Here's how the part is built. I have some questions about the finished solid (model axes, mm). Face numbers are marked on the shaded views. A direction names the side the tool comes from. Coordinates: 2 decimals unless noted, no trailing zeros. Write each loop counter-clockwise with the first axis right and the second up, starting at its lowest first coordinate (ties: lowest second). Pieces come first, ordered by that corner, then holes.
Item 1: I want a section at B-B (z = 113.5). Please give me the cut outline in (x, y), and give its area (3 significant figures).
Item 2: If we mould it in two halves opening along Z, with no side actions, what happens to the marked faces 3 and 4? For each: pulls with the +Z half, pulls with the -Z half, needs draft (parallel to the pull), parting line crosses it, or undercut.
Item 3: I want a section at A-A (x = 6.5). Please give me the cut outline in (y, z), and give its area (3 significant figures).
Item 4: I want a section at C-C (y = -5). Please give me the cut outline in (x, z) (3 decimals).
Item 5: I'm going to push flat-ended pins straight in: P1, Ø8, axis at x = -12.5, y = -5, coming from the -Z side; P2, Ø1.5, axis at x = -13.5, z = 116.5, coming from the +Y side; P3, Ø10.5, axis at x = 3.5, z = 127, coming from the +Y side; P4, Ø1.3, axis at y = -1, z = 110, coming from the -X side. Where does each tip first touch, or does it pass through?
Item 6: Please list where these lines run through material, in increasing order: line 1 (Z direction, x = -8.68, y = -11.1); line 2 (Y direction, x = -6, z = 143); line 3 (X direction, y = -0.5, z = 44.5).
Item 7: For the marked faces 1 and 2, which set-ups out of +Z, -Z, +X, -X, +Y, -Y let a thin tool reach every point of the face, with its end or its side?
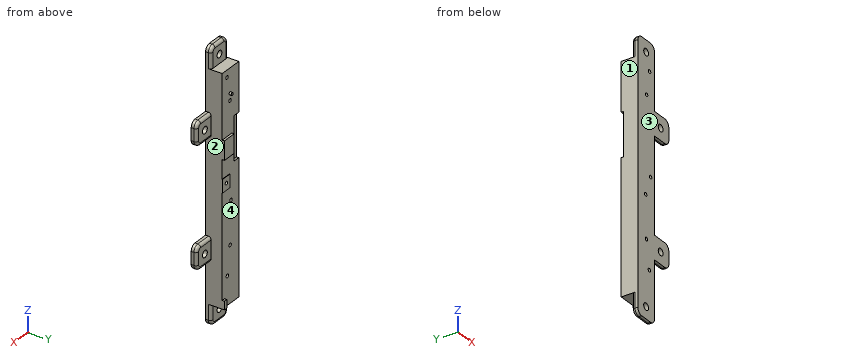
from build123d import *

# Parameters (mm, degrees)
SKETCH1_R           = 1
SKETCH1_R_2         = 1.25
SKETCH1_W           = 10.1
SKETCH1_H           = 13.47
SKETCH1_W_2         = 2.5
SKETCH1_H_2         = 6
SKETCH1_W_3         = 5.08
SKETCH1_H_3         = 31.36
BOSS_EXTRUDE1_DEPTH = 12
SKETCH1_3_W         = 10.1
SKETCH1_3_H         = 13.47
SKETCH1_3_W_2       = 2.5
SKETCH1_3_H_2       = 6
SKETCH1_3_R         = 1
BOSS_EXTRUDE2_DEPTH = 1.6
SKETCH1_4_W         = 5.08
SKETCH1_4_H         = 31.36
CUT_EXTRUDE1_DEPTH  = 1.6
BOSS_EXTRUDE3_START = 0.3
SKETCH2_W           = 7.8
SKETCH2_H           = 9.45
SKETCH2_R           = 1.25
BOSS_EXTRUDE3_DEPTH = 0.3
SKETCH3_W           = 17.3
SKETCH3_H           = 4
BOSS_EXTRUDE4_DEPTH = 15
SKETCH4_W           = 17.3
SKETCH4_H           = 4
BOSS_EXTRUDE5_DEPTH = 15
SKETCH5_W           = 17
SKETCH5_H           = 4
BOSS_EXTRUDE6_DEPTH = 15
FILLET1_R           = 4
FILLET2_R           = 2
CUT_EXTRUDE2_REACH  = 180.5
SKETCH6_R           = 2.5


with BuildPart() as part:
    # Sketch1 → Boss-Extrude1 (new body)
    # profile 1 of 5: a face of its own
    with BuildSketch(Plane(origin=(0, 0, 0), x_dir=(1, 0, 0), z_dir=(0, 1, 0))):
        Polygon((-2.5, -6), (-2.5, 0), (-17.3, 0), (-17.3, -96.08), (-12.22, -96.08), (-12.22, -127.44), (-17.3, -127.44), (-17.3, -162.4), (0, -162.4), (0, -116.51), (-10.1, -116.51), (-10.1, -103.04), (0, -103.04), (0, -6), align=None)
        with Locations((-8.115, -144.895)):
            Circle(SKETCH1_R, mode=Mode.SUBTRACT)
        with Locations(Location((-5.05, -157.28, 0), (0, 0, 270))):
            Circle(SKETCH1_R_2, mode=Mode.SUBTRACT)
        with Locations(Location((-8.115, -139.85, 0), (0, 0, 270))):
            Circle(SKETCH1_R_2, mode=Mode.SUBTRACT)
        with Locations(Location((-3.95, -85.02, 0), (0, 0, 270))):
            Circle(SKETCH1_R_2, mode=Mode.SUBTRACT)
        with Locations(Location((-9.115, -70.745, 0), (0, 0, 270))):
            Circle(SKETCH1_R_2, mode=Mode.SUBTRACT)
        with Locations(Location((-8.25, -40.21, 0), (0, 0, 270))):
            Circle(SKETCH1_R_2, mode=Mode.SUBTRACT)
        with Locations(Location((-5.3, -20.3, 0), (0, 0, 270))):
            Circle(SKETCH1_R_2, mode=Mode.SUBTRACT)
    # profile 2 of 5: a face of its own
    with BuildSketch(Plane(origin=(0, 0, 0), x_dir=(1, 0, 0), z_dir=(0, 1, 0))):
        with Locations((-5.05, -109.775)):
            Rectangle(SKETCH1_W, SKETCH1_H)
    # profile 3 of 5: a face of its own
    with BuildSketch(Plane(origin=(0, 0, 0), x_dir=(1, 0, 0), z_dir=(0, 1, 0))):
        with Locations((-1.25, -3)):
            Rectangle(SKETCH1_W_2, SKETCH1_H_2)
    # profile 4 of 5: a face of its own
    with BuildSketch(Plane(origin=(0, 0, 0), x_dir=(1, 0, 0), z_dir=(0, 1, 0))):
        with Locations((-14.76, -111.76)):
            Rectangle(SKETCH1_W_3, SKETCH1_H_3)
    # profile 5 of 5: a face of its own
    with BuildSketch(Plane(origin=(0, 0, 0), x_dir=(1, 0, 0), z_dir=(0, 1, 0))):
        with Locations((-8.115, -144.895)):
            Circle(SKETCH1_R)
    extrude(amount=-BOSS_EXTRUDE1_DEPTH)

    # Sketch1<3> → Boss-Extrude2 (add)
    with BuildSketch(Plane(origin=(0, 0, 0), x_dir=(1, 0, 0), z_dir=(0, 1, 0))):
        with Locations((-5.05, -109.775)):
            Rectangle(SKETCH1_3_W, SKETCH1_3_H)
        with Locations((-1.25, -3)):
            Rectangle(SKETCH1_3_W_2, SKETCH1_3_H_2)
        with Locations(Location((-8.115, -144.895, 0), (0, 0, 270))):
            Circle(SKETCH1_3_R)
    extrude(amount=BOSS_EXTRUDE2_DEPTH)

    # Sketch1<4> → Cut-Extrude1 (cut)
    with BuildSketch(Plane(origin=(0, 0, 0), x_dir=(1, 0, 0), z_dir=(0, 1, 0))):
        with Locations((-14.76, -111.76)):
            Rectangle(SKETCH1_4_W, SKETCH1_4_H)
    extrude(amount=-CUT_EXTRUDE1_DEPTH, mode=Mode.SUBTRACT)

    # Sketch2 → Boss-Extrude3 (add)
    with BuildSketch(Plane(origin=(0, 0, 0), x_dir=(1, 0, 0), z_dir=(0, 1, 0)).offset(BOSS_EXTRUDE3_START)):
        with Locations((-3.9, -84.835)):
            Rectangle(SKETCH2_W, SKETCH2_H)
        with Locations(Location((-3.95, -85.02, 0), (0, 0, 270))):
            Circle(SKETCH2_R, mode=Mode.SUBTRACT)
    extrude(amount=-BOSS_EXTRUDE3_DEPTH)

    # Sketch3 → Boss-Extrude4 (add)
    with BuildSketch(Plane.XY.offset(162.4)):
        with Locations((-8.65, -10)):
            Rectangle(SKETCH3_W, SKETCH3_H)
    extrude(amount=BOSS_EXTRUDE4_DEPTH)

    # Sketch4 → Boss-Extrude5 (add)
    with BuildSketch(Plane(origin=(0, 0, 0), x_dir=(-1, 0, 0), z_dir=(0, 0, -1))):
        with Locations((8.65, -10)):
            Rectangle(SKETCH4_W, SKETCH4_H)
    extrude(amount=BOSS_EXTRUDE5_DEPTH)

    # Sketch5 → Boss-Extrude6 (add)
    with BuildSketch(Plane(origin=(0, 0, 0), x_dir=(0, 0, -1), z_dir=(1, 0, 0))):
        with Locations((-123.9, -10)):
            Rectangle(SKETCH5_W, SKETCH5_H)
        with Locations((-38.5, -10)):
            Rectangle(SKETCH5_W, SKETCH5_H)
    extrude(amount=BOSS_EXTRUDE6_DEPTH)

    # Fillet1
    fillet1_edges = [part.edges().sort_by_distance(p)[0] for p in [
        (-17.3, -10, -15),
        (0, -10, -15),
        (15, -10, 132.4),
        (15, -10, 115.4),
        (15, -10, 47),
        (15, -10, 30),
        (0, -10, 177.4),
        (-17.3, -10, 177.4),
    ]]
    fillet(fillet1_edges, radius=FILLET1_R)

    # Fillet2
    fillet2_edges = [part.edges().sort_by_distance(p)[0] for p in [
        (-8.65, -8, -15),
        (-17.3, -8, -5.5),
        (-1.171572875, -8, -13.828427125),
        (-16.128427125, -8, -13.828427125),
        (-17.3, -8, 167.9),
        (15, -8, 38.5),
        (5.5, -8, 47),
        (5.5, -8, 30),
        (13.828427125, -8, 45.828427125),
        (13.828427125, -8, 31.171572875),
        (15, -8, 123.9),
        (5.5, -8, 132.4),
        (5.5, -8, 115.4),
        (13.828427125, -8, 131.228427125),
        (13.828427125, -8, 116.571572875),
        (-8.65, -8, 177.4),
        (-1.171572875, -8, 176.228427125),
        (-16.128427125, -8, 176.228427125),
    ]]
    fillet(fillet2_edges, radius=FILLET2_R)

    # Sketch6 → Cut-Extrude2 (cut, up to next)
    with BuildSketch(Plane(origin=(0, -8, 0), x_dir=(1, 0, 0), z_dir=(0, 1, 0)), mode=Mode.PRIVATE) as cut_extrude2_sk1:
        with Locations(Location((-8.68, 6.5, 0), (0, 0, 180))):
            Circle(SKETCH6_R)
    cut_extrude2_tool1 = extrude(cut_extrude2_sk1.sketch, amount=-CUT_EXTRUDE2_REACH, mode=Mode.PRIVATE) & part.part
    # Sketch6 → Cut-Extrude2 (cut, up to next)
    with BuildSketch(Plane(origin=(0, -8, 0), x_dir=(1, 0, 0), z_dir=(0, 1, 0)), mode=Mode.PRIVATE) as cut_extrude2_sk2:
        with Locations(Location((6.5, -38.5, 0), (0, 0, 180))):
            Circle(SKETCH6_R)
    cut_extrude2_tool2 = extrude(cut_extrude2_sk2.sketch, amount=-CUT_EXTRUDE2_REACH, mode=Mode.PRIVATE) & part.part
    # Sketch6 → Cut-Extrude2 (cut, up to next)
    with BuildSketch(Plane(origin=(0, -8, 0), x_dir=(1, 0, 0), z_dir=(0, 1, 0)), mode=Mode.PRIVATE) as cut_extrude2_sk3:
        with Locations(Location((6.5, -123.9, 0), (0, 0, 180))):
            Circle(SKETCH6_R)
    cut_extrude2_tool3 = extrude(cut_extrude2_sk3.sketch, amount=-CUT_EXTRUDE2_REACH, mode=Mode.PRIVATE) & part.part
    # Sketch6 → Cut-Extrude2 (cut, up to next)
    with BuildSketch(Plane(origin=(0, -8, 0), x_dir=(1, 0, 0), z_dir=(0, 1, 0)), mode=Mode.PRIVATE) as cut_extrude2_sk4:
        with Locations(Location((-8.68, -168.9, 0), (0, 0, 180))):
            Circle(SKETCH6_R)
    cut_extrude2_tool4 = extrude(cut_extrude2_sk4.sketch, amount=-CUT_EXTRUDE2_REACH, mode=Mode.PRIVATE) & part.part
    add(cut_extrude2_tool1.solids().sort_by_distance((-8.68, -8, -6.5))[0], mode=Mode.SUBTRACT)
    add(cut_extrude2_tool2.solids().sort_by_distance((6.5, -8, 38.5))[0], mode=Mode.SUBTRACT)
    add(cut_extrude2_tool3.solids().sort_by_distance((6.5, -8, 123.9))[0], mode=Mode.SUBTRACT)
    add(cut_extrude2_tool4.solids().sort_by_distance((-8.68, -8, 168.9))[0], mode=Mode.SUBTRACT)


solid = part.part
Answer:
1. outline: (-17.3, -12) - (0, -12) - (0, 1.6) - (-10.1, 1.6) - (-10.1, 0) - (-12.22, 0) - (-12.22, -1.6) - (-17.3, -1.6) - close
1. area: 216 mm2
2. face 3: needs draft
2. face 4: undercut
3. outline: (-12, 30) - (-10, 30) arc R2 ccw to (-8, 32) - (-8, 36) - (-12, 36) - close; (-12, 41) - (-8, 41) - (-8, 45) arc R2 ccw to (-10, 47) - (-12, 47) - close; (-12, 115.4) - (-10, 115.4) arc R2 ccw to (-8, 117.4) - (-8, 121.4) - (-12, 121.4) - close; (-12, 126.4) - (-8, 126.4) - (-8, 130.4) arc R2 ccw to (-10, 132.4) - (-12, 132.4) - close
3. area: 92.6 mm2
4. outline: (-17.3, 0) - (0, 0) - (0, 162.4) - (-17.3, 162.4) - close; hole circle Ø2.5 at (-9.115, 70.745); hole circle Ø2.5 at (-8.25, 40.21); hole circle Ø2.5 at (-8.115, 139.85); hole circle Ø2.5 at (-5.3, 20.3); hole circle Ø2.5 at (-5.05, 157.28); hole circle Ø2.5 at (-3.95, 85.02)
5. P1: stops at z = -14.73
5. P2: stops at y = -1.6
5. P3: stops at y = 0
5. P4: stops at x = -17.3
6. line 1: z = -15 to -9, -4 to 39.04, 41.38 to 69.57, 71.92 to 138.73, 140.97 to 166.4, 171.4 to 177.4
6. line 2: y = -12 to 0
6. line 3: x = -17.3 to 0
7. face 1: +Z, -Z, -X, +Y, -Y
7. face 2: +X, +Y
